Autodesk Inventor part; units mm, degrees
ref_plane "km_XY" through (6, 0, 0) normal (1, 0, 0) x (0, 0, -1)
ref_plane "km_YZ" through (6, 0, 0) normal (0, 0, -1) x (0, 1, 0)
ref_plane "km_ZX" through (6, 0, 0) normal (0, 1, 0) x (1, 0, 0)
sketch "Sketch_3" plane through (0, 0, 0) normal (0, 0, 1) x (1, 0, 0)
  line L0 (68, 0) -> (-68, 0)
  line L1 (0, 10) -> (0.5415, 9.4585)
  line L2 (0.5415, 9.4585) -> (5.4585, 9.4585)
  line L3 (5.4585, 9.4585) -> (6, 10)
  line L4 (6, 10) -> (6, 15)
  arc A0 (6, 15) -> (5, 16) centre (5, 15) ccw
  line L5 (5, 16) -> (1.7321, 16)
  line L6 (1.7321, 16) -> (0, 13)
  line L7 (0, 13) -> (0, 10)
revolve "Revolution1" add sketch "Sketch_3" angle 360 about axis through (68, 0, 0) along (-1, 0, 0)
thread "Thread1"
sketch "Sketch_6" plane through (0, 0, 0) normal (1, 0, 0) x (0, 1, 0)
  circle A0 centre (0, 0) radius 32
  line L0 (2, 20.9045) -> (2, 13.8745)
  line L1 (2, 13.8745) -> (-2, 13.8745)
  line L2 (-2, 13.8745) -> (-2, 20.9045)
  arc A1 (-2, 20.9045) -> (-20.9045, 2) centre (0, 0) ccw
  line L3 (-20.9045, 2) -> (-13.8745, 2)
  line L4 (-13.8745, 2) -> (-13.8745, -2)
  line L5 (-13.8745, -2) -> (-20.9045, -2)
  arc A2 (-20.9045, -2) -> (-2, -20.9045) centre (0, 0) ccw
  line L6 (-2, -20.9045) -> (-2, -13.8745)
  line L7 (-2, -13.8745) -> (2, -13.8745)
  line L8 (2, -13.8745) -> (2, -20.9045)
  arc A3 (2, -20.9045) -> (20.9045, -2) centre (0, 0) ccw
  line L9 (20.9045, -2) -> (13.8745, -2)
  line L10 (13.8745, -2) -> (13.8745, 2)
  line L11 (13.8745, 2) -> (20.9045, 2)
  arc A4 (20.9045, 2) -> (2, 20.9045) centre (0, 0) ccw
extrude "Extrusion1" cut sketch "Sketch_6" along normal blind 12
ref_plane "km_XY" through (6, 0, 0) normal (1, 0, 0) x (0, 0, -1)
ref_plane "km_YZ" through (6, 0, 0) normal (0, 0, -1) x (0, 1, 0)
ref_plane "km_ZX" through (6, 0, 0) normal (0, 1, 0) x (1, 0, 0)
ref_plane "km2_XY" through (6, 0, 0) normal (1, 0, 0) x (0, 0, -1)
ref_plane "km2_YZ" through (6, 0, 0) normal (0, 0, -1) x (0, 1, 0)
ref_plane "km2_ZX" through (6, 0, 0) normal (0, 1, 0) x (1, 0, 0)
ref_plane "ln_XY" through (0, 0, 0) normal (0, 1, 0) x (1, 0, 0)
ref_plane "ln_YZ" through (0, 0, 0) normal (1, 0, 0) x (0, 0, -1)
ref_plane "ln_ZX" through (0, 0, 0) normal (0, 0, -1) x (0, 1, 0)
ref_plane "nut_XY" through (0, 0, 0) normal (1, 0, 0) x (0, 0, -1)
ref_plane "nut_YZ" through (0, 0, 0) normal (0, 0, -1) x (0, 1, 0)
ref_plane "nut_ZX" through (0, 0, 0) normal (0, 1, 0) x (1, 0, 0)
properties part number "KM 4"
Read the model definition and answer for the solid it produces. Units are mm, in the model's axes. A direction names the side the tool comes from. Give positions to 0.01 mm unless a question says otherwise; leave off trailing zeros. Order: outer loops, then holes, each group sorted by start corner. A loop starts at its lowest first (then second) coordinate and runs counter-clockwise, first axis right, second up. Notation, with made-up numbers: (-13, -21) -> (29, -21) arc R23 cw to (29, 17) -> close; hole circle Ø7 at (-9.5, 80.5). An arc over 180 degrees is marked (long way). One line per item, written item: value. Start each with the question number.
(1) The part is cut by section B-B (x = 3.5). Determine the outline of the cut face in (y, z), and give its area (3 significant figures).
(2) A tool of negligible diameter and unlimited length cuts with its end or side. For faces 1 (the flat face through (3, 15, 2)), 2 (the flat face through (3, -15, -2)), 3 (the flat face through (3, -2, 15)), 4 (the cylindrical face through (3.343, 11.418, -11.209)), 5 (the flat face through (3, 0, -13.874)), from which of +Z, -Z, +X, -X, +Y, -Y can it reach the whole face along a straight path? Write none if from no direction.
(3) For a pull along Y with two mould halves and no side action, classify faces 6 (the flat face through (3, 2, 15)), 7 (the flat face through (3, -15, 2)), 8 (the flat face through (3, 2, -15)), 9 (the cylindrical face through (3.343, 11.209, 11.418)) as released by +Y, released by -Y, zero draft, split by the parting line, or undercut.
(4) The part is cut by section A-A (y = 0). Determine the outline of the cut face in (x, z), and give its area (3 significant figures).
(5) Flat-ended cylindrical pins translate along their axes: P1, Ø0.6, axis at x = 3, y = -14.5, coming from the -Z side; P2, Ø1.6, axis at x = 4, z = 15, coming from the -Y side; P3, Ø1.6, axis at x = 4, z = -15, coming from the +Y side. Find the tip coordinate at first contact, or state that the pin passes through.
(6) Straight lines are drawn through the part: L1, parallel to Z at x = 3.35, y = 0; L2, parallel to Y at x = 4.25, z = 5. For each, find the intervals that lie inside material, in ascending order.
Taken from the geometry:
1. outline: (-15.87, -2) arc R16 ccw to (-2, -15.87) -> (-2, -13.87) -> (2, -13.87) -> (2, -15.87) arc R16 ccw to (15.87, -2) -> (13.87, -2) -> (13.87, 2) -> (15.87, 2) arc R16 ccw to (2, 15.87) -> (2, 13.87) -> (-2, 13.87) -> (-2, 15.87) arc R16 ccw to (-15.87, 2) -> (-13.87, 2) -> (-13.87, -2) -> close; hole circle Ø18.92 at (0, 0)
1. area: 490 mm^2
2. face 1: +X, -X, +Y
2. face 2: +X, -X, -Y
2. face 3: +Z, +X, -X
2. face 4: -Z, +X, -X, +Y
2. face 5: -Z, +X, -X
3. face 6: undercut
3. face 7: zero draft
3. face 8: undercut
3. face 9: released by +Y
4. outline: (0, -13) -> (0.5, -13.87) -> (6, -13.87) -> (6, -10) -> (5.46, -9.46) -> (0.54, -9.46) -> (0, -10) -> close; (0, 10) -> (0.54, 9.46) -> (5.46, 9.46) -> (6, 10) -> (6, 13.87) -> (0.5, 13.87) -> (0, 13) -> close
4. area: 52.0 mm^2
5. P1: z = -7.37
5. P2: y = -7.37
5. P3: y = 7.37
6. L1: -13.87 to -9.46, 9.46 to 13.87
6. L2: -15.2 to -8.03, 8.03 to 15.2
